from build123d import *

# Parameters (mm, degrees)
F0_W      = 103.75
F0_H      = 64.5
F1_DEPTH  = 2.2
F2_T      = -1.9
F3_W      = 26.5
F3_H      = 15
F4_DEPTH  = 12.7
F5_R      = 2
F6_R      = 2
F7_W      = 4.9
F7_H      = 60.7
F8_DEPTH  = 2.5
F9_W      = 4.9
F9_H      = 60.7
F10_DEPTH = 2.5
F11_R     = 0.8
F12_DEPTH = 25.4
F13_R     = 0.8
F14_DEPTH = 25.4
F15_R     = 0.8
F16_DEPTH = 25.4
F17_R     = 0.8
F18_DEPTH = 25.4


with BuildPart() as f1:
    # F0 (on Top) → F1 (new body, symmetric)
    with BuildSketch(Plane.XY):
        Rectangle(F0_W, F0_H)
    extrude(amount=F1_DEPTH, both=True)

    # F2
    f2_openings = [f1.faces().sort_by_distance(p)[0] for p in [
        (0, 0, 2.2),
    ]]
    offset(amount=F2_T, openings=f2_openings)

    # F3 (on Top) → F4 (cut, symmetric)
    with BuildSketch(Plane.XY):
        Rectangle(F3_W, F3_H)
    extrude(amount=F4_DEPTH, both=True, mode=Mode.SUBTRACT)

    # F5
    f5_edges = [f1.edges().sort_by_distance(p)[0] for p in [
        (-51.875, 32.25, 0),
    ]]
    fillet(f5_edges, radius=F5_R)

    # F6
    f6_edges = [f1.edges().sort_by_distance(p)[0] for p in [
        (-51.875, -32.25, 0),
        (51.875, -32.25, 0),
        (51.875, 32.25, 0),
    ]]
    fillet(f6_edges, radius=F6_R)

    # F7 (on face) → F8 (join)
    with BuildSketch(Plane.XY.offset(-0.3)):
        with Locations((-47.525, 0)):
            Rectangle(F7_W, F7_H)
    extrude(amount=F8_DEPTH)

    # F9 (on face) → F10 (join)
    with BuildSketch(Plane.XY.offset(-0.3)):
        with Locations((47.525, 0)):
            Rectangle(F9_W, F9_H)
    extrude(amount=F10_DEPTH)

    # F11 (on face) → F12 (cut)
    with BuildSketch(Plane.XY.offset(2.2)):
        with Locations((49.875, -30.25)):
            Circle(F11_R)
    extrude(amount=-F12_DEPTH, mode=Mode.SUBTRACT)

    # F13 (on face) → F14 (cut)
    with BuildSketch(Plane.XY.offset(2.2)):
        with Locations((49.875, 30.25)):
            Circle(F13_R)
    extrude(amount=-F14_DEPTH, mode=Mode.SUBTRACT)

    # F15 (on face) → F16 (cut)
    with BuildSketch(Plane.XY.offset(2.2)):
        with Locations((-49.875, -30.25)):
            Circle(F15_R)
    extrude(amount=-F16_DEPTH, mode=Mode.SUBTRACT)

    # F17 (on face) → F18 (cut)
    with BuildSketch(Plane.XY.offset(2.2)):
        with Locations((-49.875, 30.25)):
            Circle(F17_R)
    extrude(amount=-F18_DEPTH, mode=Mode.SUBTRACT)


solid = f1.part
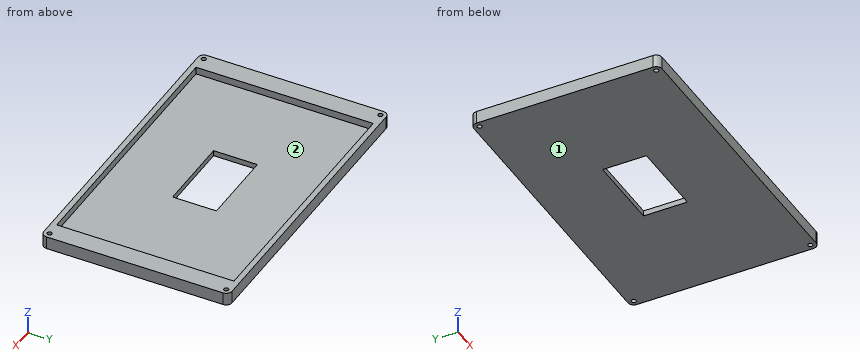
Can you work these out from the model? Positions are in its coordinate system, mm. Face numbers are marked on the shaded views. Give positions to 0.01 mm unless a question says otherwise; leave off trailing zeros. Write each loop counter-clockwise with the first axis right and the second up, starting at its lowest first coordinate (ties: lowest second). Pieces come first, ordered by that corner, then holes. Notation, with made-up numbers: (12, -17.5) -> (48, -17.5) arc R25 ccw to (48, 15.5) -> close; hole circle Ø7 at (59, 33.5). An arc over 180 degrees is marked (long way). Answer as a JSON object with one key per item and string values. Group by question number.
Item 1: Suppose I cut it at A-A (y = 0). Please give me the cut outline in (x, z) (3 decimals).
Item 2: We'd pull the mould along X, two halves only. Please class the marked faces 1 and 2: +X half, -X half, draft (parallel to the pull), parting line (faces both ways), or undercut.
Item 3: I'm going to push flat-ended pins straight in: P1, Ø1.4, axis at x = 49.875, y = 30.25, coming from the -Z side; P2, Ø3, axis at x = -10.5, y = 15, coming from the +Z side. Where does each tip first touch, or does it pass through?
Item 4: Suppose I cut it at B-B (z = 0.45). Please give me the cut outline in (x, y) (3 decimals), plus the area to 3 significant figures.
Item 5: Please list where these lines run through material, in increasing order: line 1 (Y direction, x = -39, z = 1.85); line 2 (X direction, y = 21, z = 0.7) (3 decimals); line 3 (Z direction, x = 22.5, y = 13.5). Write a range as [from, to].
Item 6: Suppose I cut it at D-D (y = 20.5). Please give me the cut outline in (x, z) (3 decimals).
Item 7: Suppose I cut it at C-C (x = -39). Please give me the cut outline in (y, z).
Findings:
{
 "1": {"outline": "(-51.875, -2.2) -> (-13.25, -2.2) -> (-13.25, -0.3) -> (-45.075, -0.3) -> (-45.075, 2.2) -> (-51.875, 2.2) -> close; (13.25, -2.2) -> (51.875, -2.2) -> (51.875, 2.2) -> (45.075, 2.2) -> (45.075, -0.3) -> (13.25, -0.3) -> close"},
 "2": {"face 1": "draft", "face 2": "undercut"},
 "3": {"P1": "passes through", "P2": "stops at z = -0.3"},
 "4": {"outline": "(-51.875, -30.25) arc R2 ccw to (-49.875, -32.25) -> (49.875, -32.25) arc R2 ccw to (51.875, -30.25) -> (51.875, 30.25) arc R2 ccw to (49.875, 32.25) -> (-49.875, 32.25) arc R2 ccw to (-51.875, 30.25) -> close; hole circle Ø1.6 at (-49.875, -30.25); hole circle Ø1.6 at (-49.875, 30.25); hole (-45.075, -30.35) -> (45.075, -30.35) -> (45.075, 30.35) -> (-45.075, 30.35) -> close; hole circle Ø1.6 at (49.875, -30.25); hole circle Ø1.6 at (49.875, 30.25)", "area": "1,210 mm²"},
 "5": {"line 1": "y = [-32.25, -30.35], [30.35, 32.25]", "line 2": "x = [-51.875, -45.075], [45.075, 51.875]", "line 3": "z = [-2.2, -0.3]"},
 "6": {"outline": "(-51.875, -2.2) -> (51.875, -2.2) -> (51.875, 2.2) -> (45.075, 2.2) -> (45.075, -0.3) -> (-45.075, -0.3) -> (-45.075, 2.2) -> (-51.875, 2.2) -> close"},
 "7": {"outline": "(-32.25, -2.2) -> (32.25, -2.2) -> (32.25, 2.2) -> (30.35, 2.2) -> (30.35, -0.3) -> (-30.35, -0.3) -> (-30.35, 2.2) -> (-32.25, 2.2) -> close"}
}
